from build123d import *

# Parameters (mm, degrees)
F1_DEPTH = 939.8
F2_W     = 95.7861989737
F2_H     = 17.2806475312
F3_DEPTH = 153.6309794951
F4_R     = 46.1278485026
F5_DEPTH = 44.9828275762


with BuildPart() as f1:
    # F0 (on Right) → F1 (new body)
    with BuildSketch(Plane.YZ):
        Polygon((-16.2542276084, 49.0534752607), (-40.6355895102, 0), (107.4585616589, -47.2123473883), (26.1873789132, 23.1404751539), align=None)
    extrude(amount=F1_DEPTH)

    # F2 (on face) → F3 (cut, through all)
    with BuildSketch(Plane(origin=(0, -32.5854994089, 16.1961787542), x_dir=(1, 0, 0), z_dir=(0, -0.8954862226, 0.4450892328))):
        with Locations((135.2553740144, 8.6403237656)):
            Rectangle(F2_W, F2_H)
    extrude(amount=-F3_DEPTH, mode=Mode.SUBTRACT)

    # F4 (on face) → F5 (cut, through all)
    with BuildSketch(Plane(origin=(0, -3.7489093909, -11.7594566838), x_dir=(1, 0, 0), z_dir=(0, -0.3037380425, -0.9527555833))):
        with Locations((275.9448885918, -41.0455577075)):
            Circle(F4_R)
    extrude(amount=F5_DEPTH, mode=Mode.SUBTRACT)


solid = f1.part
Verification items for the finished model (mm, model axes). A direction names the side the tool comes from. Give positions to 0.01 mm unless a question says otherwise; leave off trailing zeros. Order: outer loops, then holes, each group sorted by start corner. A loop starts at its lowest first (then second) coordinate and runs counter-clockwise, first axis right, second up. Notation, with made-up numbers: M 71.25,52 L 87.25,52 A22 cw 87.25,63 Z; hole C 5.25,25 d8. An arc over 180 degrees is marked long. Answer as a JSON object with one key per item and string values. Group by question number.
1) Depth check by flat-ended pin: pin 1 Ø3 at (x, y) = (642.5, 24) entering from -Z; pin 2 Ø10 at (x, z) = (196.5, 19.5) entering from +Y; pin 3 Ø1.5 at (x, z) = (468, 1) entering from +Y. Enter the tip coordinate at first touch or a pass-through.
2) Scan lines: line 1 along Y through (x, z) = (144, 3); line 2 along Y through (x, z) = (268, 17.5); line 3 along Z through (x, y) = (492, 87). Record each from-to range of solid material in increasing order. Write a range as [from, to].
3) Access from +Z, -Z, +X, -X, +Y, -Y to the whole of each face (thin tool, end or side, straight path). Record for faces 1 (the face through (134.585, 22.837, 7.947)), 2 (the face through (463.321, 67.392, -12.528)).
4) Cross-section at A-A (y = 9). Enter the section's corners in (x, z).
5) Cross-section at B-B (y = 45). Enter the section's corners in (x, z), then the cut area to 3 significant figures.
6) Cross-section at C-C (x = 391.5). Enter the section's corners in (y, z), then the cut area to 3 significant figures.
7) Mould release check, pull along Z, two halves, no side actions. Record for faces 3 (the face through (134.58, 19.31, -9.6)), 4 (the face through (463.32, 5.26, 35.92)), 5 (the face through (939.8, 17, -2)), 6 (the face through (87.362, 24, -2)): released by +Z, released by -Z, zero draft, split by the parting line, or undercut.
Result sheet:
{
 "1": {"pin 1": "stops at z = -21.08", "pin 2": "stops at y = 36.17", "pin 3": "stops at y = 52.63"},
 "2": {"line 1": "y = [-39.14, -6.04], [32.79, 49.45]", "line 2": "y = [-31.94, 32.7]", "line 3": "z = [-40.69, -29.5]"},
 "3": {"face 1": "none", "face 2": "+Z, +X, -X, +Y"},
 "4": {"outline": "M 0,-15.82 L 939.8,-15.82 L 939.8,33.63 L 0,33.63 Z; hole M 87.36,-4.47 L 183.15,-4.47 L 183.15,14.82 L 87.36,14.82 Z"},
 "5": {"outline": "M 0,-27.3 L 939.8,-27.3 L 939.8,6.86 L 0,6.86 Z; hole M 87.36,-22.37 L 183.15,-22.37 L 183.15,-3.07 L 87.36,-3.07 Z", "area": "30,300 mm2"},
 "6": {"outline": "M -40.64,0 L 107.46,-47.21 L 26.19,23.14 L -16.25,49.05 Z", "area": "4,650 mm2"},
 "7": {"face 3": "undercut", "face 4": "released by +Z", "face 5": "zero draft", "face 6": "undercut"}
}
